Geometry: final body of the model. Coordinates: model frame, mm. A direction names the side the tool comes from. Give positions to 0.01 mm unless a question says otherwise; leave off trailing zeros. Write each loop counter-clockwise with the first axis right and the second up, starting at its lowest first coordinate (ties: lowest second). Pieces come first, ordered by that corner, then holes. Notation, with made-up numbers: (1.25, -26.5) - (44.25, -26.5) arc R15 ccw to (44.25, 1.5) - close; hole circle Ø5 at (38, -3.75). An arc over 180 degrees is marked (long way). Use CSV: the item, a comma, the result in double quotes. Start each with the question number.
(1) Section C-C on x = 229.5. Output: boundary loops of the cut face in (y, z).
(2) Section D-D on z = 174.5. Output: boundary loops of the cut face in (x, y), and give its area (3 significant figures).
(3) Section B-B on z = 514. Output: boundary loops of the cut face in (x, y), and give its area (3 significant figures).
(4) First-contact query: pin 1 Ø6 at (x, z) = (43, 156.5) entering from -Y; pin 2 Ø1.5 at (x, y) = (-274.5, 86.5) entering from -Z; pin 3 Ø1.5 at (x, z) = (362.5, 196.5) entering from -Y. Flat tips, straight axial feed; report the tip coordinate or a pass-through.
(5) Section A-A on y = 296. Output: boundary loops of the cut face in (x, z), and give its area (3 significant figures).
(6) Line query: probe 1 along Y at (x, z) = (43, 57.5); probe 2 along Z at (x, y) = (-135, 407); probe 3 along X at (y, z) = (308.5, 54.5). Output: solid intervals per line, ascending. Write a range as [from, to].
(7) Draft query along X for faces 1 (the flat face through (4, 0, 562)), 2 (the flat face through (418.033, 188.557, 295.834)), 3 (the flat face through (647.7, 225, 340)). Return one class per face: released by +X, released by -X, zero draft, split by the parting line, or undercut.
(8) Reachability of faces 4 (the flat face through (11, 444.5, 296)), 5 (the flat face through (458, 25.4, 76)), 6 (the flat face through (57, 448, 25.4)) from +Z, -Z, +X, -X, +Y, -Y: full face, straight path, thin tool, end or side. Return the list, or none.
from build123d import *

# Parameters (mm, degrees)
F1_DEPTH = 457.2
F3_DEPTH = 25.4
F5_DEPTH = 638.23027


with BuildPart() as f1:
    # F0 (on Front) → F1 (new body)
    with BuildSketch(Plane.XZ):
        Polygon((-622.3, 25.4), (-469.9, 25.4), (-317.5, 558.8), (342.9, 558.8), (495.3, 25.4), (647.7, 25.4), (647.7, 663.63027), (-622.3, 663.63027), align=None)
    extrude(amount=-F1_DEPTH)

    # F2 (on face) → F3 (join)
    with BuildSketch(Plane.XZ):
        Polygon((444.5, 25.4), (495.3, 25.4), (444.5, 203.2), align=None)
    extrude(amount=-F3_DEPTH)

    # F4 (on face) → F5 (join, through all)
    with BuildSketch(Plane.XY.offset(663.63027)):
        Polygon((495.3, 457.2), (-469.9, 457.2), (-469.9, 330.2), (-136.640207, 444.5), (162.040207, 444.5), (495.3, 330.2), align=None)
    extrude(amount=-F5_DEPTH)


solid = f1.part
Check values:
1,outline,"(0, 558.8) - (421.36, 558.8) - (421.36, 25.4) - (457.2, 25.4) - (457.2, 663.63) - (0, 663.63) - close"
2,outline,"(-622.3, 0) - (-427.3, 0) - (-427.3, 344.81) - (-136.64, 444.5) - (162.04, 444.5) - (452.7, 344.81) - (452.7, 25.4) - (444.5, 25.4) - (444.5, 0) - (647.7, 0) - (647.7, 457.2) - (-622.3, 457.2) - close"
2,area,"219,000 mm²"
3,outline,"(-622.3, 0) - (-330.3, 0) - (-330.3, 378.08) - (-136.64, 444.5) - (162.04, 444.5) - (355.7, 378.08) - (355.7, 0) - (647.7, 0) - (647.7, 457.2) - (-622.3, 457.2) - close"
3,area,"289,000 mm²"
4,pin 1,"stops at y = 444.5"
4,pin 2,"stops at z = 558.8"
4,pin 3,"stops at y = 375.49"
5,outline,"(-622.3, 25.4) - (-469.9, 25.4) - (-317.5, 558.8) - (342.9, 558.8) - (495.3, 25.4) - (647.7, 25.4) - (647.7, 663.63) - (-622.3, 663.63) - close"
5,area,"377,000 mm²"
6,probe 1,"y = [444.5, 457.2]"
6,probe 2,"z = [558.8, 663.63]"
6,probe 3,"x = [-622.3, -461.59], [486.99, 647.7]"
7,face 1,"zero draft"
7,face 2,"undercut"
7,face 3,"released by +X"
8,face 4,"-Z, -Y"
8,face 5,"-Z"
8,face 6,"-Z, +X, -X, +Y, -Y"
